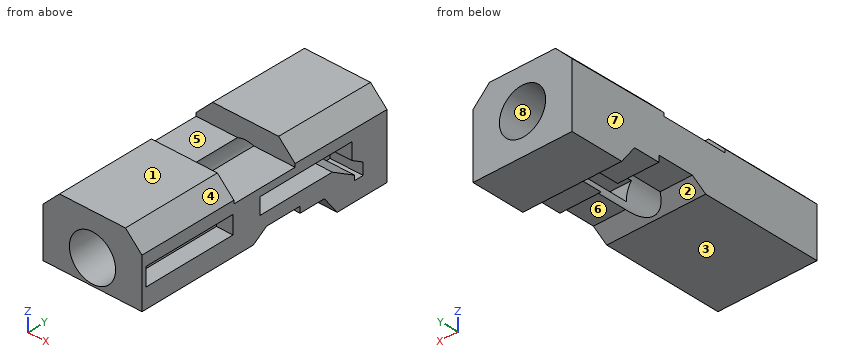
```python
from build123d import *

# Parameters (mm, degrees)
F1_DEPTH  = 76.2
F3_DEPTH  = 127
F4_SIZE   = 12.7
F5_R      = 17.78
F5_R_2    = 12.7
F6_DEPTH  = 254
F8_DEPTH  = 25.4
F9_W      = 72.165888
F9_H      = 13.97679
F10_DEPTH = 12.7


with BuildPart() as f1:
    # F0 (on Right) → F1 (new body)
    with BuildSketch(Plane.YZ):
        Polygon((72.027118, 67.494695), (-131.172882, 68.619423), (-131.172882, -34.105305), (72.027118, -34.105305), align=None)
    extrude(amount=F1_DEPTH)

    # F2 (on face) → F3 (cut)
    with BuildSketch(Plane.YZ.offset(76.2)):
        Polygon((-38.896065, 11.837486), (-131.172882, 11.837486), (-131.172882, -34.105305), (72.027118, -34.105305), (72.027118, 0), (30.702649, 0), (20.148747, 14.404653), (0, 14.404653), (0, 19.253744), (-27.771682, 19.253744), align=None)
        Polygon((-131.172882, 68.619423), (-131.172882, 62.895566), (-54.972882, 62.895566), (-54.972882, 47.655566), (-4.172882, 47.655566), (-4.172882, 62.895566), (72.024081, 62.215233), (72.027118, 0), (72.027118, 67.494695), align=None)
    extrude(amount=-F3_DEPTH, mode=Mode.SUBTRACT)

    # F4
    f4_edges = [f1.edges().sort_by_distance(p)[0] for p in [
        (76.2, -93.072882, 62.895566),
        (76.2, 33.925599, 62.5554),
        (0, -93.072882, 62.895566),
        (0, 33.925599, 62.5554),
    ]]
    chamfer(f4_edges, length=F4_SIZE)

    # F5 (on face) → F6 (cut)
    with BuildSketch(Plane.XZ.offset(131.172882)):
        with Locations((38.1, 31.016526)):
            Circle(F5_R)
        with Locations((38.1, 31.016526)):
            Circle(F5_R_2, mode=Mode.SUBTRACT)
        with Locations((38.1, 31.016526)):
            Circle(F5_R_2)
    extrude(amount=-F6_DEPTH, mode=Mode.SUBTRACT)

    # F7 (on face) → F8 (cut)
    with BuildSketch(Plane.YZ.offset(76.2)):
        Polygon((42.803339, 41.952084), (-33.396661, 41.952084), (-33.396661, 29.252084), (26.66526, 29.252084), (45.232709, 18.085102), (45.232709, 14.487018), (52.239504, 14.487018), (52.239504, 23.576912), (42.803339, 29.252084), align=None)
    extrude(amount=-F8_DEPTH, mode=Mode.SUBTRACT)

    # F9 (on face) → F10 (cut)
    with BuildSketch(Plane.YZ.offset(76.2)):
        with Locations((-91.808209, 33.943634)):
            Rectangle(F9_W, F9_H)
    extrude(amount=-F10_DEPTH, mode=Mode.SUBTRACT)


solid = f1.part
```
Geometry check sheet. Reference: the model listing, model coordinates, mm. Face numbers are marked on the shaded views. A direction names the side the tool comes from. Coordinates: 2 decimals unless noted, no trailing zeros. Loops run counter-clockwise (first coordinate to the right, second up) from the corner with the lowest first, then second, coordinate; pieces in that order, holes last.
Item 1: Sectioned sample at A-A, the plane y = -6.5. Record the boundary of the cut face in (x, z), then the cut area to 3 significant figures.
Item 2: Sectioned sample at D-D, the plane x = 38.1. Record the boundary of the cut face in (y, z).
Item 3: Release check for a two-part mould opening along X. For the marked faces 6, 7 and 8 record: released by +X, released by -X, zero draft, split by the parting line, or undercut.
Item 4: Sectioned sample at B-B, the plane z = 34.5. Record the boundary of the cut face in (x, y), then the cut area to 3 significant figures.
Item 5: Go/stop test with flat-tipped pins: pin 1 Ø2 at (y, z) = (-83.5, 28) entering from +X; pin 2 Ø10 at (x, y) = (56.5, -99) entering from -Z; pin 3 Ø6 at (x, y) = (62.5, 10.5) entering from -Z. Record where each tip stops, or that it passes through.
Item 6: Sectioned sample at C-C, the plane x = 47. Record the boundary of the cut face in (y, z).
Item 7: Thickness scan on line 1 (Y direction, x = 72, z = 33); line 2 (Y direction, x = 46, z = 54.5); line 3 (X direction, y = 63, z = 27.5). Record the ranges inside material, lowest first.
Item 8: Access from +Z, -Z, +X, -X, +Y, -Y to the whole of each face (thin tool, end or side, straight path). Record for the marked faces 1, 2, 3, 4 and 5.
Check result:
1. outline: (0, 19.25) - (24.77, 19.25) arc R17.78 cw to (31.83, 47.66) - (0, 47.66) - close; (44.37, 47.66) arc R17.78 cw to (52.12, 41.95) - (76.2, 41.95) - (76.2, 47.66) - close; (51.43, 19.25) - (76.2, 19.25) - (76.2, 29.25) - (55.79, 29.25) arc R17.78 cw to start
1. area: 1,020 mm2
2. outline: (-131.17, 11.84) - (-38.9, 11.84) - (-36.8, 13.24) - (-131.17, 13.24) - close; (-131.17, 48.8) - (-54.97, 48.8) - (-54.97, 62.9) - (-131.17, 62.9) - close; (-4.17, 48.8) - (72.02, 48.8) - (72.02, 62.22) - (-4.17, 62.9) - close; (21, 13.24) - (30.7, 0) - (72.03, 0) - (72.03, 13.24) - close
3. face 6: zero draft
3. face 7: released by -X
3. face 8: undercut
4. outline: (0, -131.17) - (20.66, -131.17) - (20.66, 72.03) - (0, 72.03) - close; (55.54, -131.17) - (76.2, -131.17) - (76.2, -127.89) - (63.5, -127.89) - (63.5, -55.73) - (76.2, -55.73) - (76.2, -33.4) - (55.54, -33.4) - close; (55.54, 42.8) - (76.2, 42.8) - (76.2, 72.03) - (55.54, 72.03) - close
4. area: 5,910 mm2
5. pin 1: stops at x = 63.5
5. pin 2: stops at z = 11.84
5. pin 3: stops at z = 14.4
6. outline: (-131.17, 11.84) - (-38.9, 11.84) - (-33.22, 15.62) - (-131.17, 15.62) - close; (-131.17, 46.41) - (72.02, 46.41) - (72.02, 62.22) - (-4.17, 62.9) - (-4.17, 47.66) - (-54.97, 47.66) - (-54.97, 62.9) - (-131.17, 62.9) - close; (0, 14.4) - (20.15, 14.4) - (30.7, 0) - (72.03, 0) - (72.03, 15.62) - (0, 15.62) - close
7. line 1: y = -131.17 to -127.89, -55.73 to -33.4, 42.8 to 72.03
7. line 2: y = -131.17 to -54.97, -4.17 to 72.02
7. line 3: x = 0 to 20.67, 55.53 to 76.2
8. face 1: +Z, +X, -X, +Y, -Y
8. face 2: -Z, +X, -X
8. face 3: -Z, +X, -X, -Y
8. face 4: +Z, +X, +Y, -Y
8. face 5: +Z, +X, -X
